Build history of the part. All positions in model axes, mm. Face numbers are marked on the shaded views. A direction names the side the tool comes from. Round coordinates to 2 decimals unless told otherwise and drop trailing zeros. Order: outer loops, then holes, each group sorted by start corner. A loop starts at its lowest first (then second) coordinate and runs counter-clockwise, first axis right, second up. Notation, with made-up numbers: M -23,65 L 24,65 A31 ccw 24,89 Z; hole C 58,-25.5 d11. An arc over 180 degrees is marked long. One line per item, written item: value. Start each with the question number.
Item 1: Probe L1, parallel to X at y = 6.5, z = 3; L2, parallel to Y at x = 36, z = 0.5; L3, parallel to Y at x = 15.5, z = 10.25. List the from-to ranges inside material, lowest first.
Item 2: Band-saw the part on B-B, the plane y = 11.75. Give the number of separate pieces and of enclosed holes in the cut face, then the cut area to 3 significant figures.
Item 3: Band-saw the part on A-A, the plane z = 11.5. Write the cut outline in (x, y), then the cut area to 3 significant figures.
Item 4: Pin check, flat tips, straight feed: pin 1 (6 mm diameter, centred on x = 46.5, z = 19, fed in from -Y); pin 2 (5.5 mm diameter, centred on x = 12.5, z = 8.5, fed in from +Y); pin 3 (4 mm diameter, centred on x = 4, y = 5, fed in from +Z); pin 4 (3 mm diameter, centred on x = 45, y = 10.5, fed in from -Z). Stop position of each tip, or through.
Item 5: Band-saw the part on C-C, the plane z = 3.25. Write the cut outline in (x, y).
Item 6: Two-plate mould, pull along X, no slides. Class the marked faces 1, 2, 3 and 4: +X half, -X half, draft (parallel to the pull), parting line (faces both ways), or undercut.
Item 7: Tool access for the marked faces 5, 6 and 7: list every direction of +Z, -Z, +X, -X, +Y, -Y with a clear straight run to the whole face (end or side of a thin tool).
Item 8: Band-saw the part on D-D, the plane y = 5. Write the cut outline in (x, z), then the cut area to 3 significant figures.
Autodesk Inventor part; units mm, degrees
ref_plane "YZ Plane" through (0, 0, 0) normal (1, 0, 0) x (0, 1, 0)
ref_plane "XZ Plane" through (0, 0, 0) normal (0, 1, 0) x (-1, 0, 0)
ref_plane "XY Plane" through (0, 0, 0) normal (0, 0, 1) x (1, 0, 0)
sketch "Sketch1" plane through (0, 0, 0) normal (0, 0, 1) x (1, 0, 0)
  line L0 (0, 0) -> (40, 0)
  line L1 (40, 0) -> (40, 10)
  line L2 (40, 10) -> (0, 10)
  line L3 (0, 10) -> (0, 0)
  circle A0 centre (4, 5) radius 1.6
  circle A1 centre (36, 5) radius 1.6
  line L4 (0, 0) -> (-12, 0)
  line L5 (-12, 0) -> (-12, 13)
  line L6 (-12, 13) -> (0, 13)
  line L7 (0, 13) -> (0, 0)
  line L8 (40, 0) -> (52, 0)
  line L9 (52, 0) -> (52, 13)
  line L10 (52, 13) -> (40, 13)
  line L11 (40, 13) -> (40, 0)
  point P0 (0, 5)
  dimension "d0" = 40
  dimension "d1" = 10
  dimension "d22" = 3.2
  dimension "d23" = 3.2
  dimension "d24" = 4
  dimension "d25" = 4
  dimension "d43" = 12
  dimension "d44" = 12
  dimension "d45" = 13
  dimension "d46" = 13
extrude "Extrusion1" add sketch "Sketch1" along normal blind 5 contours L3 L2 L1 L0
extrude "Extrusion5" add sketch "Sketch1" along normal blind 5 contours L4 L5 L6 L7 L3 | L1 L11 L10 L9 L8
sketch "Sketch2" plane through (0, 0, 5) normal (0, 0, 1) x (1, 0, 0)
  line L0 (40, 10) -> (0, 10)
  line L1 (0, 0) -> (40, 0)
  line L2 (7.5, 10) -> (32.5, 10)
  line L3 (32.5, 10) -> (32.5, 6)
  line L4 (32.5, 6) -> (7.5, 6)
  line L5 (7.5, 6) -> (7.5, 10)
  line L6 (7.5, 0) -> (32.5, 0)
  line L7 (32.5, 0) -> (32.5, 4)
  line L8 (32.5, 4) -> (7.5, 4)
  line L9 (7.5, 4) -> (7.5, 0)
  line L10 (0, 13) -> (-12, 13)
  line L11 (52, 13) -> (40, 13)
  line L12 (-12, 13) -> (0, 13)
  line L13 (0, 13) -> (0, 10)
  line L14 (0, 10) -> (-12, 10)
  line L15 (-12, 10) -> (-12, 13)
  line L16 (52, 13) -> (40, 13)
  line L17 (40, 13) -> (40, 10)
  line L18 (40, 10) -> (52, 10)
  line L19 (52, 10) -> (52, 13)
  point P0 (20, 10)
  point P1 (20, 10)
  point P2 (20, 0)
  point P3 (20, 0)
  dimension "d14" = 25
  dimension "d15" = 25
  dimension "d31" = 2
  dimension "d32" = 4
  dimension "d33" = 4
extrude "Extrusion2" add sketch "Sketch2" along normal blind 13 contours L3 L4 L5 L0 | L9 L8 L7 L1
fillet "Fillet1" radius 1 2 edges at (20, 6, 18) (20, 4, 18)
sketch "Sketch3" plane through (0, 0, 5) normal (0, 0, 1) x (1, 0, 0)
  circle A0 centre (4, 5) radius 1.6
  circle A1 centre (36, 5) radius 1.6
  line L0 (6.75, 6.5877) -> (6.75, 3.4123)
  line L1 (6.75, 3.4123) -> (4, 1.8246)
  line L2 (4, 1.8246) -> (1.25, 3.4123)
  line L3 (1.25, 3.4123) -> (1.25, 6.5877)
  line L4 (1.25, 6.5877) -> (4, 8.1754)
  line L5 (4, 8.1754) -> (6.75, 6.5877)
  line L6 (33.25, 6.5877) -> (36, 8.1754)
  line L7 (36, 8.1754) -> (38.75, 6.5877)
  line L8 (38.75, 6.5877) -> (38.75, 3.4123)
  line L9 (38.75, 3.4123) -> (36, 1.8246)
  line L10 (36, 1.8246) -> (33.25, 3.4123)
  line L11 (33.25, 3.4123) -> (33.25, 6.5877)
  point P0 (0, 0)
  dimension "d39" = 5.5
  dimension "d40" = 5.5
extrude "Extrusion3" cut sketch "Sketch3" against normal blind 3
sketch "Sketch4" plane through (0, 0, 5) normal (0, 0, 1) x (1, 0, 0)
  line L0 (7.5, 6) -> (7.5, 10)
  line L1 (32.5, 4) -> (32.5, 0)
  line L2 (7.5, 6) -> (32.5, 6)
  line L3 (32.5, 6) -> (32.5, 4)
  line L4 (32.5, 4) -> (7.5, 4)
  line L5 (7.5, 4) -> (7.5, 6)
  point P0 (0, 0)
extrude "Extrusion4" add sketch "Sketch4" along normal blind 4
extrude "Extrusion7" add sketch "Sketch2" along normal blind 20 contours L13 L14 L15 L10 | L19 L18 L17 L11
sketch "Sketch5" plane through (-12, 10, 5) normal (0, -1, 0) x (1, 0, 0)
  circle A0 centre (6, 16) radius 1.6
  circle A1 centre (58, 16) radius 1.6
  line L0 (0, 20) -> (12, 20)
  line L1 (52, 20) -> (64, 20)
  point P0 (15, -5)
  point P1 (6, 20)
  point P2 (58, 20)
  dimension "d49" = 3.2
  dimension "d50" = 3.2
  dimension "d56" = 4
extrude "Extrusion6" cut sketch "Sketch5" against normal blind 5
chamfer "Chamfer2" distance 3 angle 45 2 edges at (-6, 10, 5) (46, 10, 5)
fillet "Fillet2" radius 6 4 edges at (0, 11.5, 25) (-12, 11.5, 25) (40, 11.5, 25) (52, 11.5, 25)
equation "\"d23\" = d22"
equation "\"d44\" = d43"
equation "\"d45\" = d46"
equation "\"d15\" = d14"
equation "\"d32\" = d33"
equation "\"d40\" = d39"
equation "\"d50\" = d49"
properties part number "GT2 grip v2"
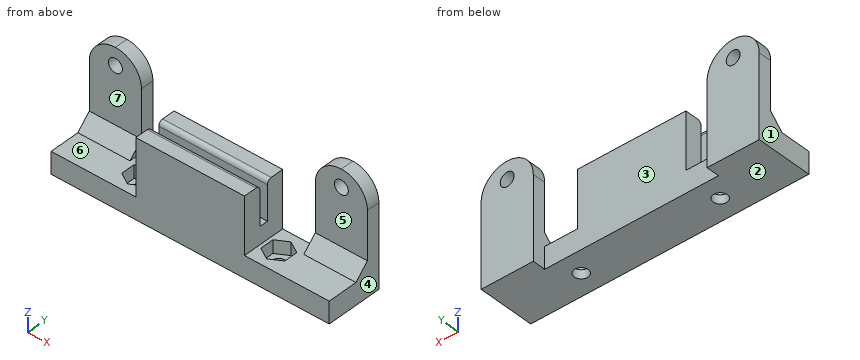
Output:
1. L1: x = -12 to 1.25, 6.75 to 33.25, 38.75 to 52
1. L2: y = 0 to 3.4, 6.6 to 10
1. L3: y = 0 to 4, 6 to 10
2. separate pieces: 2
2. enclosed holes: 2
2. area: 553 mm²
3. outline: M -12,10 L 0,10 L 0,13 L -12,13 Z; M 7.5,0 L 32.5,0 L 32.5,4 L 7.5,4 Z; M 7.5,6 L 32.5,6 L 32.5,10 L 7.5,10 Z; M 40,10 L 52,10 L 52,13 L 40,13 Z
3. area: 272 mm²
4. pin 1: stops at y = 10
4. pin 2: stops at y = 10
4. pin 3: stops at z = 2
4. pin 4: stops at z = 0
5. outline: M -12,0 L 52,0 L 52,13 L 40,13 L 40,10 L 0,10 L 0,13 L -12,13 Z; hole M 1.25,3.41 L 4,1.82 L 6.75,3.41 L 6.75,6.59 L 4,8.18 L 1.25,6.59 Z; hole M 33.25,3.41 L 36,1.82 L 38.75,3.41 L 38.75,6.59 L 36,8.18 L 33.25,6.59 Z
6. face 1: -X half
6. face 2: draft
6. face 3: undercut
6. face 4: +X half
7. face 5: +Z, +X, -Y
7. face 6: +Z, -Y
7. face 7: +Z, -X, -Y
8. outline: M -12,0 L 2.4,0 L 2.4,2 L 1.25,2 L 1.25,5 L -12,5 Z; M 5.6,0 L 34.4,0 L 34.4,2 L 33.25,2 L 33.25,5 L 32.5,5 L 32.5,9 L 7.5,9 L 7.5,5 L 6.75,5 L 6.75,2 L 5.6,2 Z; M 37.6,0 L 52,0 L 52,5 L 38.75,5 L 38.75,2 L 37.6,2 Z
8. area: 374 mm²
